Design review of the part built by this model. Coordinates are the model's own, in mm. A direction names the side the tool comes from. Give positions to 0.01 mm unless a question says otherwise; leave off trailing zeros. Write each loop counter-clockwise with the first axis right and the second up, starting at its lowest first coordinate (ties: lowest second). Pieces come first, ordered by that corner, then holes. Notation, with made-up numbers: (71.5, 75) -> (95.5, 75) arc R22 cw to (95.5, 109) -> close; hole circle Ø2 at (-15.5, 31.25). An arc over 180 degrees is marked (long way). Return JSON: item names as keys, results as strings. Group by question number.
from build123d import *

# Parameters (mm, degrees)
SKETCH2_R           = 2
BOSS_EXTRUDE1_DEPTH = 1
SKETCH3_R           = 1.5
BOSS_EXTRUDE2_DEPTH = 3
SKETCH4_R           = 2.25
BOSS_EXTRUDE3_DEPTH = 0.5
SKETCH5_R           = 1.45
BOSS_EXTRUDE4_DEPTH = 5
CHAMFER3_SIZE       = 0.25


with BuildPart() as part:
    # Sketch2 → Boss-Extrude1 (new body)
    with BuildSketch(Plane(origin=(0, 0, 0), x_dir=(1, 0, 0), z_dir=(0, 1, 0))):
        with Locations(Location((0, 0, 0), (0, 0, 270))):
            Circle(SKETCH2_R)
    extrude(amount=BOSS_EXTRUDE1_DEPTH)

    # Sketch3 → Boss-Extrude2 (add)
    with BuildSketch(Plane(origin=(0, 1, 0), x_dir=(1, 0, 0), z_dir=(0, 1, 0))):
        with Locations(Location((0, 0, 0), (0, 0, 270))):
            Circle(SKETCH3_R)
    extrude(amount=BOSS_EXTRUDE2_DEPTH)

    # Sketch4 → Boss-Extrude3 (add)
    with BuildSketch(Plane(origin=(0, 4, 0), x_dir=(1, 0, 0), z_dir=(0, 1, 0))):
        with Locations(Location((0, 0, 0), (0, 0, 270))):
            Circle(SKETCH4_R)
    extrude(amount=BOSS_EXTRUDE3_DEPTH)

    # Sketch5 → Boss-Extrude4 (add)
    with BuildSketch(Plane(origin=(0, 4.5, 0), x_dir=(1, 0, 0), z_dir=(0, 1, 0))):
        with Locations(Location((0, 0, 0), (0, 0, 270))):
            Circle(SKETCH5_R)
    extrude(amount=BOSS_EXTRUDE4_DEPTH)

    # Chamfer3
    chamfer3_edges = [part.edges().sort_by_distance(p)[0] for p in [
        (0, 9.5, -1.45),
    ]]
    chamfer(chamfer3_edges, length=CHAMFER3_SIZE)


solid = part.part
Q1. Tool access review of faces 1 (the face through (-1.952, 0.493, -0.434)), 2 (the face through (0.06, 6.84, -1.45)), 3 (the face through (0, 4, -2)), 4 (the face through (0.676, 4.246, 2.146)): name each direction out of +Z, -Z, +X, -X, +Y, -Y from which nothing blocks a thin tool from reaching the whole face with its end or side.
Q2. Insertion check: pin 1 (2 mm diameter, centred on y = 8.5, z = 0.5, fed in from -X). The pin has a flat end and moves straight along its axis. Give the tip position at first contact, or say it passes through.
Q3. Mouldability with a two-part tool opening along Y and no side actions: class faces 5 (the face through (0, 0, 0)), 6 (the face through (0.45, 2.48, 1.43)), 7 (the face through (0, 9.5, 0)) as +Y half, -Y half, draft (parallel to the pull), parting line (faces both ways), or undercut.
Q4. Take a section at D-D, the plane y = 8.5. Give the boundary of the cut face in (x, z).
Q5. Take a section at C-C, the plane x = 0. Give the boundary of the cut face in (y, z).
Q6. Take a section at B-B, the plane z = 0. Give the boundary of the cut face in (x, y), plus the area to 3 significant figures.
Q7. Take a section at A-A, the plane x = 1.65. Give the boundary of the cut face in (y, z), plus the area to 3 significant figures.
Q8. For L1, parallel to Y at x = 1.85, z = 0.2; L2, parallel to Y at x = 1.5, z = 1.4; L3, parallel to Z at x = -0.65, y = 8, list the stretches that pass through material, from the lowest coordinate up. Write a range as from..to.
Final values:
{
 "1": {"face 1": "-Y", "face 2": "+Y", "face 3": "none", "face 4": "+Y, -Y"},
 "2": {"pin 1": "stops at x = -1.45"},
 "3": {"face 5": "-Y half", "face 6": "undercut", "face 7": "+Y half"},
 "4": {"outline": "circle Ø2.9 at (0, 0)"},
 "5": {"outline": "(0, -2) -> (1, -2) -> (1, -1.5) -> (4, -1.5) -> (4, -2.25) -> (4.5, -2.25) -> (4.5, -1.45) -> (9.25, -1.45) -> (9.5, -1.2) -> (9.5, 1.2) -> (9.25, 1.45) -> (4.5, 1.45) -> (4.5, 2.25) -> (4, 2.25) -> (4, 1.5) -> (1, 1.5) -> (1, 2) -> (0, 2) -> close"},
 "6": {"outline": "(-2.25, 4) -> (-1.5, 4) -> (-1.5, 1) -> (-2, 1) -> (-2, 0) -> (2, 0) -> (2, 1) -> (1.5, 1) -> (1.5, 4) -> (2.25, 4) -> (2.25, 4.5) -> (1.45, 4.5) -> (1.45, 9.25) -> (1.2, 9.5) -> (-1.2, 9.5) -> (-1.45, 9.25) -> (-1.45, 4.5) -> (-2.25, 4.5) -> close", "area": "29.7 mm²"},
 "7": {"outline": "(0, -1.13) -> (1, -1.13) -> (1, 1.13) -> (0, 1.13) -> close; (4, -1.53) -> (4.5, -1.53) -> (4.5, 1.53) -> (4, 1.53) -> close", "area": "3.79 mm²"},
 "8": {"L1": "y = 0..1, 4..4.5", "L2": "y = 4..4.5", "L3": "z = -1.3..1.3"}
}
